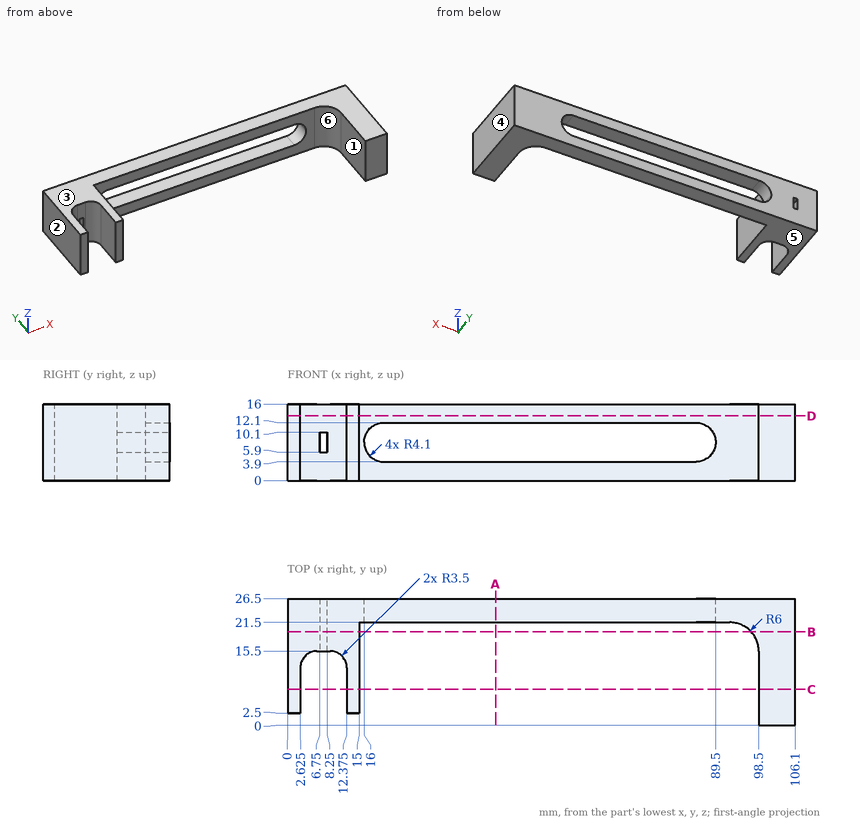
For this review, use the dimensioned drawing (mm, ordinates from the lowest corner) and the shaded views. A direction names the side the tool comes from. Round coordinates to 2 decimals unless told otherwise and drop trailing zeros. Loops run counter-clockwise (first coordinate to the right, second up) from the corner with the lowest first, then second, coordinate; pieces in that order, holes last. Notation, with made-up numbers: M -7.5,85.25 L 37.5,85.25 A32 cw 37.5,120.25 Z; hole C -21,-27 d4. An arc over 180 degrees is marked long. Answer as a JSON object with one key per item and string values.
(1) Draft analysis for pull direction X (two halves, no side actions). For the marked faces 1, 2, 3 and 4, state which applies: released by +X, released by -X, zero draft, split by the parting line, or undercut.
Resolved:
{"face 1": "undercut", "face 2": "released by -X", "face 3": "zero draft", "face 4": "released by +X"}
(2) Tool access review of the marked faces 5 and 6: name each direction out of +Z, -Z, +X, -X, +Y, -Y from which nothing blocks a thin tool from reaching the whole face with its end or side.
Resolved:
{"face 5": "-Z, +X, -X, +Y, -Y", "face 6": "+Z, -Z, -Y"}
(3) Take a section at C-C on y = 7.5. Give the boundary of the cut face in (x, z) (3 decimals).
Resolved:
{"outline": "M 0,0 L 2.625,0 L 2.625,16 L 0,16 Z; M 12.375,0 L 15,0 L 15,16 L 12.375,16 Z; M 98.5,0 L 106.1,0 L 106.1,16 L 98.5,16 Z"}
(4) Take a section at A-A on x = 43.5. Give the boundary of the cut face in (y, z).
Resolved:
{"outline": "M 21.5,0 L 26.5,0 L 26.5,3.9 L 21.5,3.9 Z; M 21.5,12.1 L 26.5,12.1 L 26.5,16 L 21.5,16 Z"}
(5) To check wall thickness, follow line 1 along X through (y, z) = (8, 7.5) (3 decimals); line 2 along Y through (x, z) = (23.5, 12.75); line 3 along X through (y, z) = (13.75, 14). State the ranges of each line that lie inside material, in increasing order.
Resolved:
{"line 1": "0 to 2.625, 12.375 to 15, 98.5 to 106.1", "line 2": "21.5 to 26.5", "line 3": "0 to 3.09, 11.91 to 15, 98.5 to 106.1"}
(6) Clearance check with flat-ended pins moving along their axes: P1, Ø2, axis at x = 13, z = 8, coming from the -Y side; P2, Ø1, axis at x = 23.5, z = 4.5, coming from the +Y side; P3, Ø0.8, axis at x = 7, z = 9, coming from the -Y side. State where each tip first meets the part, or that it passes through.
Resolved:
{"P1": "y = 2.5", "P2": "through", "P3": "y = 15.5"}
(7) Take a section at B-B on y = 19.5. Give the boundary of the cut face in (x, z).
Resolved:
{"outline": "M 0,0 L 15,0 L 15,16 L 0,16 Z; M 96.97,0 L 106.1,0 L 106.1,16 L 96.97,16 Z; hole M 6.75,5.9 L 8.25,5.9 L 8.25,10.1 L 6.75,10.1 Z"}
(8) Take a section at D-D on z = 13.5. Give the boundary of the cut face in (x, y) (3 decimals).
Resolved:
{"outline": "M 0,2.5 L 2.625,2.5 L 2.625,12 A3.5 cw 6.125,15.5 L 8.875,15.5 A3.5 cw 12.375,12 L 12.375,2.5 L 15,2.5 L 15,21.5 L 92.5,21.5 A6 cw 98.5,15.5 L 98.5,0 L 106.1,0 L 106.1,26.5 L 0,26.5 Z"}
